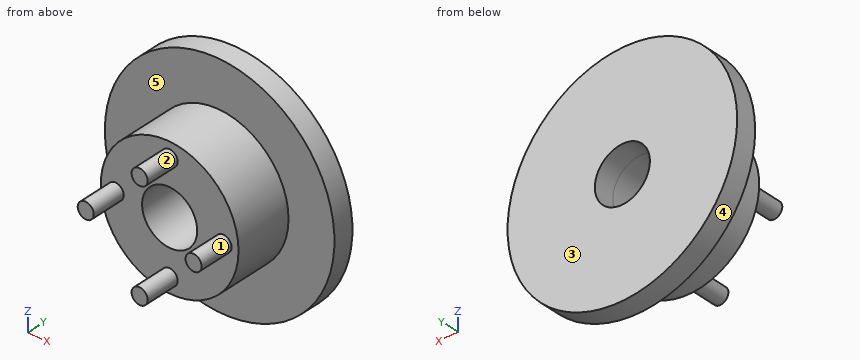
from build123d import *

# Parameters (mm, degrees)
F0_R     = 15
F0_R_2   = 6
F1_DEPTH = 12.5
F3_R     = 25
F3_R_2   = 6
F4_DEPTH = 4.5
F5_R     = 1.75
F6_DEPTH = 7.5


with BuildPart() as f1:
    # F0 (on Front) → F1 (new body)
    with BuildSketch(Plane.XZ):
        Circle(F0_R)
        Circle(F0_R_2, mode=Mode.SUBTRACT)
    extrude(amount=F1_DEPTH)

    # F3 (on face) → F4 (join)
    with BuildSketch(Plane(origin=(0, 0, 0), x_dir=(-1, 0, 0), z_dir=(0, 1, 0))):
        Circle(F3_R)
        Circle(F3_R_2, mode=Mode.SUBTRACT)
    extrude(amount=F4_DEPTH)

    # F5 (on face) → F6 (join)
    with BuildSketch(Plane.XZ.offset(12.5)):
        with Locations((0, 11.741299)):
            Circle(F5_R)
        with Locations((-11.741299, 0)):
            Circle(F5_R)
        with Locations((11.741299, 0)):
            Circle(F5_R)
        with Locations((0, -11.741299)):
            Circle(F5_R)
    extrude(amount=F6_DEPTH)


solid = f1.part
For this review, take the finished solid that the model builds, in its own axes (mm). Face numbers are marked on the shaded views. A direction names the side the tool comes from. Round coordinates to 2 decimals unless told otherwise and drop trailing zeros. Write each loop counter-clockwise with the first axis right and the second up, starting at its lowest first coordinate (ties: lowest second). Pieces come first, ordered by that corner, then holes. Notation, with made-up numbers: M -35,-7.75 L 20,-7.75 A3 cw 20,-2.75 Z; hole C 44.5,6 d11. An arc over 180 degrees is marked long. Write item = value, one per line. Start each with the question number.
(1) For the marked faces 4 and 5, list the 3-axis set-ups (+Z, -Z, +X, -X, +Y, -Y) from which the entire face can be reached by the end or side of a thin tool; tool diameter is ignored.
(2) We need section A-A (x = 0). Give the boundary of the cut face in (y, z), then the cut area to 4 significant figures.
(3) For line 1 along Z through (x, y) = (0, 1.65); line 2 along Z through (x, y) = (4, -9.75); line 3 along X through (y, z) = (-6, 1), list the stretches that pass through material, from the lowest coordinate up.
(4) We need section B-B (z = 0). Give the boundary of the cut face in (x, y).
(5) We need section D-D (x = 7.5). Give the boundary of the cut face in (y, z), then the cut area to 3 significant figures.
(6) We need section C-C (y = -2.25). Give the boundary of the cut face in (x, z).
(7) The part is to be moulded in two halves that separate along Z. For the marked faces 1, 2 and 3, say which applies: +Z half, -Z half, draft (parallel to the pull), parting line (faces both ways), or undercut.
(8) Clearance check with flat-ended pins moving along their axes: pin 1 Ø6 at (y, z) = (-9.5, -16) entering from -X; pin 2 Ø25 at (x, z) = (0, -6.5) entering from -Y; pin 3 Ø1.5 at (y, z) = (-14, -5) entering from +X; pin 4 Ø4 at (y, z) = (-16.5, -9) entering from -X. State where each tip first meets the part, or that it passes through.
Results found:
q1.face_4 = +Y, -Y
q1.face_5 = -Y
q2.outline = M -20,-13.49 L -12.5,-13.49 L -12.5,-15 L 0,-15 L 0,-25 L 4.5,-25 L 4.5,-6 L -12.5,-6 L -12.5,-9.99 L -20,-9.99 Z; M -20,9.99 L -12.5,9.99 L -12.5,6 L 4.5,6 L 4.5,25 L 0,25 L 0,15 L -12.5,15 L -12.5,13.49 L -20,13.49 Z
q2.area = 448.5 mm²
q3.line_1 = -25 to -6, 6 to 25
q3.line_2 = -14.46 to -4.47, 4.47 to 14.46
q3.line_3 = -14.97 to -5.92, 5.92 to 14.97
q4.outline = M -25,0 L -15,0 L -15,-12.5 L -13.49,-12.5 L -13.49,-20 L -9.99,-20 L -9.99,-12.5 L -6,-12.5 L -6,4.5 L -25,4.5 Z; M 6,-12.5 L 9.99,-12.5 L 9.99,-20 L 13.49,-20 L 13.49,-12.5 L 15,-12.5 L 15,0 L 25,0 L 25,4.5 L 6,4.5 Z
q5.outline = M -12.5,-12.99 L 0,-12.99 L 0,-23.85 L 4.5,-23.85 L 4.5,23.85 L 0,23.85 L 0,12.99 L -12.5,12.99 Z
q5.area = 539 mm²
q6.outline = C 0,0 d30; hole C 0,0 d12
q7.face_1 = parting line
q7.face_2 = undercut
q7.face_3 = draft
q8.pin_1 = -7.48
q8.pin_2 = -20
q8.pin_3 = through
q8.pin_4 = -1.59
